Read the model definition and answer for the solid it produces. Units are mm, in the model's axes. A direction names the side the tool comes from. Round coordinates to 2 decimals unless told otherwise and drop trailing zeros. Loops run counter-clockwise (first coordinate to the right, second up) from the corner with the lowest first, then second, coordinate; pieces in that order, holes last. Notation, with made-up numbers: (-28, -38) -> (-12, -38) arc R6 ccw to (-12, -31) -> close; hole circle Ø4 at (-19, 55). An arc over 180 degrees is marked (long way). Put each result on its own line as item: value.
Autodesk Inventor part; units mm, degrees
ref_plane "YZ Plane" through (0, 0, 0) normal (1, 0, 0) x (0, 1, 0)
ref_plane "XZ Plane" through (0, 0, 0) normal (0, 1, 0) x (-1, 0, 0)
ref_plane "XY Plane" through (0, 0, 0) normal (0, 0, 1) x (1, 0, 0)
sketch "スケッチ1" plane through (0, 0, 0) normal (0, 1, 0) x (-1, 0, 0)
  line L0 (0, 0) -> (-15, 0)
  line L1 (-15, 0) -> (-15, 15)
  line L2 (-15, 15) -> (0, 15)
  line L3 (0, 15) -> (0, 0)
  line L4 (-1.2, 13.8) -> (-13.8, 13.8)
  line L5 (-13.8, 13.8) -> (-13.8, 1.2)
  line L6 (-13.8, 1.2) -> (-1.2, 1.2)
  line L7 (-1.2, 1.2) -> (-1.2, 13.8)
  dimension "d0" = 15
  dimension "d1" = 15
  dimension "d2" = 1.2
  dimension "d3" = 1.2
  dimension "d4" = 1.2
  dimension "d5" = 1.2
extrude "押し出し1" add sketch "スケッチ1" along normal blind 61.5
sketch "スケッチ2" plane through (0, 0, 15) normal (0, 0, 1) x (1, 0, 0)
  line L0 (0, 0) -> (0, 61.5)
  line L1 (0, 61.5) -> (15, 61.5)
  line L2 (0, 0) -> (15, 0)
  point P0 (7.5, 54)
  point P1 (7.5, 7.5)
  dimension "d8" = 7.5
  dimension "d9" = 7.5
  dimension "d10" = 7.5
  dimension "d11" = 7.5
hole "穴1" at (7.5, 54, 15) at (7.5, 7.5, 15) direction (0, 0, -1) diameter 3 end through all
sketch "スケッチ3" plane through (15, 0, 15) normal (1, 0, 0) x (0, 0, -1)
  line L0 (0, 61.5) -> (15, 61.5)
  line L1 (15, 0) -> (15, 61.5)
  point P0 (7.5, 55.5)
  point P1 (7.5, 49.5)
  point P2 (7.5, 43.5)
  point P3 (7.5, 37.5)
  point P4 (7.5, 31.5)
  point P5 (7.5, 25.5)
  point P6 (7.5, 19.5)
  point P7 (7.5, 13.5)
  point P8 (7.5, 7.5)
  dimension "d19" = 6
  dimension "d20" = 7.5
  dimension "d23" = 6
hole "穴2" at (15, 55.5, 7.5) at (15, 49.5, 7.5) at (15, 43.5, 7.5) at (15, 37.5, 7.5) at (15, 31.5, 7.5) at (15, 25.5, 7.5) at (15, 19.5, 7.5) at (15, 13.5, 7.5) at (15, 7.5, 7.5) direction (-1, 0, 0) diameter 4.5 end through all
equation "\"d3\" = d2"
equation "\"d4\" = d3"
equation "\"d5\" = d3"
properties part number "ロボットベース15x15_5" material "アルミニウム 6061"
Item 1: The part is cut by section C-C (y = 54). Determine the outline of the cut face in (x, z), then the cut area to 3 significant figures.
Derived:
outline: (0, 0) -> (6, 0) -> (6, 1.2) -> (1.2, 1.2) -> (1.2, 5.82) -> (0, 5.82) -> close; (0, 9.18) -> (1.2, 9.18) -> (1.2, 13.8) -> (6, 13.8) -> (6, 15) -> (0, 15) -> close; (9, 0) -> (15, 0) -> (15, 5.82) -> (13.8, 5.82) -> (13.8, 1.2) -> (9, 1.2) -> close; (9, 13.8) -> (13.8, 13.8) -> (13.8, 9.18) -> (15, 9.18) -> (15, 15) -> (9, 15) -> close
area: 51.0 mm^2
Item 2: Which of the six approach directions +Z, -Z, +X, -X, +Y, -Y give full straight-line access (tool end or side, diameter ignored) to faces 1 (the cylindrical face through (0.592, 27.696, 7.988)), 2 (the flat face through (13.8, 30, 5))?
Derived:
face 1: +X, -X
face 2: +Y, -Y
Item 3: For a pull along Y with two mould halves and no side action, classify faces 3 (the cylindrical face through (14.392, 21.696, 7.988)), 4 (the flat face through (0, 30, 4)), 5 (the flat face through (1, 0, 8)), 6 (the cylindrical face through (0.59, 35.27, 7.79)) as pulls with the +Y half, pulls with the -Y half, needs draft (parallel to the pull), parting line crosses it, or undercut.
Derived:
face 3: undercut
face 4: needs draft
face 5: pulls with the -Y half
face 6: undercut
Item 4: The part is cut by section B-B (x = 11.25). Determine the outline of the cut face in (y, z).
Derived:
outline: (0, 0) -> (61.5, 0) -> (61.5, 1.2) -> (0, 1.2) -> close; (0, 13.8) -> (61.5, 13.8) -> (61.5, 15) -> (0, 15) -> close
Item 5: The part is cut by section D-D (y = 19.5). Determine the outline of the cut face in (x, z), then the cut area to 3 significant figures.
Derived:
outline: (0, 0) -> (15, 0) -> (15, 5.25) -> (13.8, 5.25) -> (13.8, 1.2) -> (1.2, 1.2) -> (1.2, 5.25) -> (0, 5.25) -> close; (0, 9.75) -> (1.2, 9.75) -> (1.2, 13.8) -> (13.8, 13.8) -> (13.8, 9.75) -> (15, 9.75) -> (15, 15) -> (0, 15) -> close
area: 55.4 mm^2
Item 6: The part is cut by section A-A (z = 4.25). Determine the outline of the cut face in (x, y).
Derived:
outline: (0, 0) -> (1.2, 0) -> (1.2, 61.5) -> (0, 61.5) -> close; (13.8, 0) -> (15, 0) -> (15, 61.5) -> (13.8, 61.5) -> close
Item 7: Find the intervals of material crossed by line 1 along Y through (x, z) = (7.5, 14.55); line 2 along Z through (x, y) = (3, 57), in increasing order.
Derived:
line 1: y = 0 to 6, 9 to 52.5, 55.5 to 61.5
line 2: z = 0 to 1.2, 13.8 to 15
